Build history of the part. All positions in model axes, mm. Give positions to 0.01 mm unless a question says otherwise; leave off trailing zeros. Loops run counter-clockwise (first coordinate to the right, second up) from the corner with the lowest first, then second, coordinate; pieces in that order, holes last. Notation, with made-up numbers: (15.5, 4.25) -> (56.5, 4.25) arc R8 ccw to (56.5, 18.25) -> close; hole circle Ø11 at (-14.75, -9.75). An arc over 180 degrees is marked (long way). Answer as a JSON object with one key per item and string values. Group by question number.
Q1. Band-saw the part on D-D, the plane x = -16. Write the cut outline in (y, z), plus the area to 3 significant figures.
Q2. Wall check: probe 1 along Z at (x, y) = (0, -1.5); probe 2 along X at (y, z) = (-1.05, -1.5); probe 3 along Z at (x, y) = (14, -2.7). Give the ranges that are in metal, low to high. Write a range as from..to.
Q3. Band-saw the part on C-C, the plane y = -1.65. Write the cut outline in (x, z).
Q4. Band-saw the part on B-B, the plane z = 0. Write the cut outline in (x, y).
Q5. Band-saw the part on A-A, the plane x = 0. Write the cut outline in (y, z).
Q6. Drop flat-ended pins along their axis: pin 1 (1.5 mm diameter, centred on y = -1.5, z = -3.5, fed in from +X); pin 2 (1.5 mm diameter, centred on x = 3, y = -2.5, fed in from -Z); pin 3 (1.5 mm diameter, centred on y = -2, z = -16, fed in from +X). Give the stop position or say it passes through.
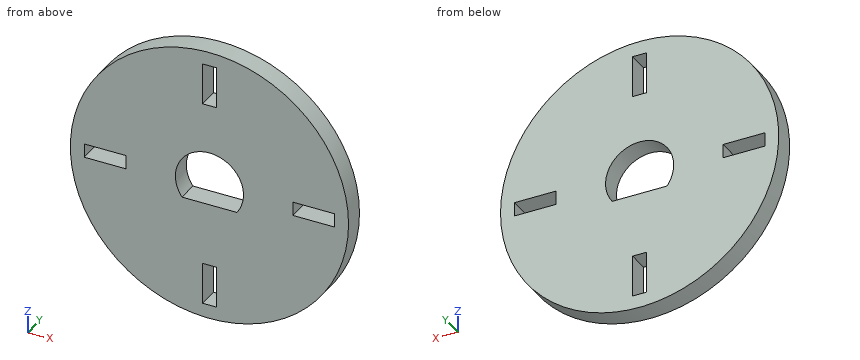
from build123d import *

# Parameters (mm, degrees)
F0_R     = 20
F1_DEPTH = 3


with BuildPart() as f1:
    # F0 (on Front) → F1 (new body)
    with BuildSketch(Plane.XZ):
        Circle(F0_R)
        Polygon((-1, -12), (0, -12), (1, -12), (1, -18), (-1, -18), align=None, mode=Mode.SUBTRACT)
        Polygon((-12, 1), (-12, 0), (-12, -1), (-18, -1), (-18, 1), align=None, mode=Mode.SUBTRACT)
        with BuildLine():
            ThreePointArc((-3.949684, -2.9), (0, 4.9), (3.949684, -2.9))
            Line((3.949684, -2.9), (-3.949684, -2.9))
        make_face(mode=Mode.SUBTRACT)
        Polygon((12, -1), (12, 0), (12, 1), (18, 1), (18, -1), align=None, mode=Mode.SUBTRACT)
        Polygon((1, 12), (0, 12), (-1, 12), (-1, 18), (1, 18), align=None, mode=Mode.SUBTRACT)
    extrude(amount=F1_DEPTH)


solid = f1.part
Worked answers:
{
 "1": {"outline": "(-3, -12) -> (0, -12) -> (0, -1) -> (-3, -1) -> close; (-3, 1) -> (0, 1) -> (0, 12) -> (-3, 12) -> close", "area": "66.0 mm2"},
 "2": {"probe 1": "-20..-18, -12..-2.9, 4.9..12, 18..20", "probe 2": "-19.94..-4.66, 4.66..19.94", "probe 3": "-14.28..-1, 1..14.28"},
 "3": {"outline": "circle Ø40 at (0, 0); hole (-18, -1) -> (-12, -1) -> (-12, 1) -> (-18, 1) -> close; hole (-3.95, -2.9) -> (3.95, -2.9) arc R4.9 ccw (long way) to start; hole (-1, -18) -> (1, -18) -> (1, -12) -> (-1, -12) -> close; hole (-1, 12) -> (1, 12) -> (1, 18) -> (-1, 18) -> close; hole (12, -1) -> (18, -1) -> (18, 1) -> (12, 1) -> close"},
 "4": {"outline": "(-20, -3) -> (-18, -3) -> (-18, 0) -> (-20, 0) -> close; (-12, -3) -> (-4.9, -3) -> (-4.9, 0) -> (-12, 0) -> close; (4.9, -3) -> (12, -3) -> (12, 0) -> (4.9, 0) -> close; (18, -3) -> (20, -3) -> (20, 0) -> (18, 0) -> close"},
 "5": {"outline": "(-3, -20) -> (0, -20) -> (0, -18) -> (-3, -18) -> close; (-3, -12) -> (0, -12) -> (0, -2.9) -> (-3, -2.9) -> close; (-3, 4.9) -> (0, 4.9) -> (0, 12) -> (-3, 12) -> close; (-3, 18) -> (0, 18) -> (0, 20) -> (-3, 20) -> close"},
 "6": {"pin 1": "x = 19.81", "pin 2": "z = -19.87", "pin 3": "x = 12.94"}
}
